```python
from build123d import *

# Parameters (mm, degrees)
F0_W     = 60
F0_H     = 60
F0_R     = 2.5
F1_DEPTH = 2


with BuildPart() as f1:
    # F0 (on Top) → F1 (new body)
    with BuildSketch(Plane.XY):
        with Locations((30, -30)):
            Rectangle(F0_W, F0_H)
        with Locations((5, -55)):
            Circle(F0_R, mode=Mode.SUBTRACT)
        Polygon((6.3547094441, -26.5316670423), (8.2590716884, -30.1279213632), (10.1760247574, -26.5316670423), (11.0809902868, -26.5316670423), (8.6808643177, -30.9337341476), (8.6808643177, -33.722601831), (7.835705206, -33.722601831), (7.835705206, -30.9730804749), (5.4403007962, -26.5316670423), align=None, mode=Mode.SUBTRACT)
        Polygon((31.1360398773, -51.5644881962), (33.3232842313, -55.0153143704), (32.4584262999, -55.0153143704), (30.6971567479, -52.1338888575), (28.9043335069, -55.0153143704), (28.0968459192, -55.0153143704), (30.2754847216, -51.5903048508), (28.2445745543, -48.46218686), (29.0879186068, -48.46218686), (30.714367851, -51.0581949129), (32.3551596812, -48.46218686), (33.1655157861, -48.46218686), align=None, mode=Mode.SUBTRACT)
        with Locations((55, -55)):
            Circle(F0_R, mode=Mode.SUBTRACT)
        with Locations((5, -5)):
            Circle(F0_R, mode=Mode.SUBTRACT)
    extrude(amount=F1_DEPTH)


solid = f1.part
```
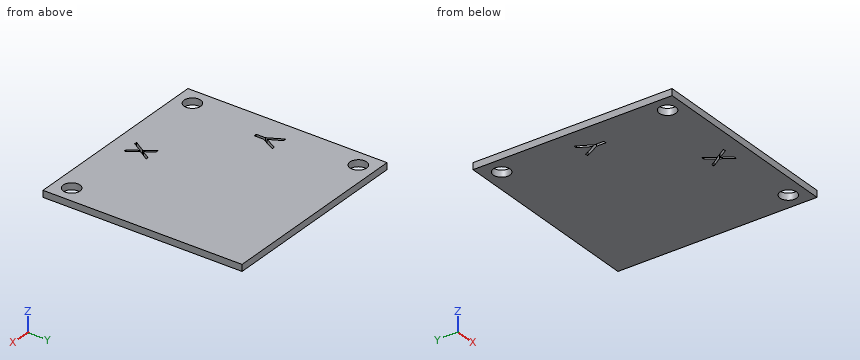
Geometry check sheet. Reference: the model listing, model coordinates, mm. Give positions to 0.01 mm unless a question says otherwise; leave off trailing zeros. Order: outer loops, then holes, each group sorted by start corner. A loop starts at its lowest first (then second) coordinate and runs counter-clockwise, first axis right, second up.
1. Section check B-B, the plane z = 1.1. Enter the section's corners in (x, y), and give its area (3 significant figures).
2. Thickness scan on L1, parallel to Y at x = 5, z = 1.9; L2, parallel to Y at x = 55, z = 0.75; L3, parallel to X at y = -27.5, z = 0.4. Record the ranges inside material, lowest first.
3. Section check A-A, the plane y = -5. Enter the section's corners in (x, z), and give its area (3 significant figures).
4. Section check C-C, the plane x = 55. Enter the section's corners in (y, z).
Values follow:
1. outline: (0, -60) - (60, -60) - (60, 0) - (0, 0) - close; hole circle Ø5 at (5, -55); hole circle Ø5 at (5, -5); hole (5.44, -26.53) - (7.84, -30.97) - (7.84, -33.72) - (8.68, -33.72) - (8.68, -30.93) - (11.08, -26.53) - (10.18, -26.53) - (8.26, -30.13) - (6.35, -26.53) - close; hole (28.1, -55.02) - (28.9, -55.02) - (30.7, -52.13) - (32.46, -55.02) - (33.32, -55.02) - (31.14, -51.56) - (33.17, -48.46) - (32.36, -48.46) - (30.71, -51.06) - (29.09, -48.46) - (28.24, -48.46) - (30.28, -51.59) - close; hole circle Ø5 at (55, -55)
1. area: 3,520 mm2
2. L1: y = -60 to -57.5, -52.5 to -7.5, -2.5 to 0
2. L2: y = -60 to -57.5, -52.5 to 0
2. L3: x = 0 to 5.96, 6.87 to 9.66, 10.55 to 60
3. outline: (0, 0) - (2.5, 0) - (2.5, 2) - (0, 2) - close; (7.5, 0) - (60, 0) - (60, 2) - (7.5, 2) - close
3. area: 110 mm2
4. outline: (-60, 0) - (-57.5, 0) - (-57.5, 2) - (-60, 2) - close; (-52.5, 0) - (0, 0) - (0, 2) - (-52.5, 2) - close
